Model file for the job. Use its own axes, mm. Give positions to 0.01 mm unless a question says otherwise; leave off trailing zeros. Order: outer loops, then holes, each group sorted by start corner. A loop starts at its lowest first (then second) coordinate and runs counter-clockwise, first axis right, second up. Notation, with made-up numbers: (51, 74.5) -> (109, 74.5) arc R19 ccw to (109, 84.5) -> close; hole circle Ø10 at (-22.5, 89.25). An arc over 180 degrees is marked (long way). Use CSV: the item, a comma, the result in double quotes. Start each with the question number.
1. Cut at A-A on y = 2. List the corners of the cut face in (x, z).
2. Wall check: line 1 (X direction, y = -15, z = 116.5); line 2 (Y direction, x = -28.5, z = 28); line 3 (Y direction, x = -27.5, z = 75). Give the ranges that are in metal, low to high. Write a range as from..to.
3. Drop a flat-ended pin along its axis: pin 1 (3 mm diameter, centred on x = 13.5, z = 142.5, fed in from +Y). Give the stop position or say it passes through.
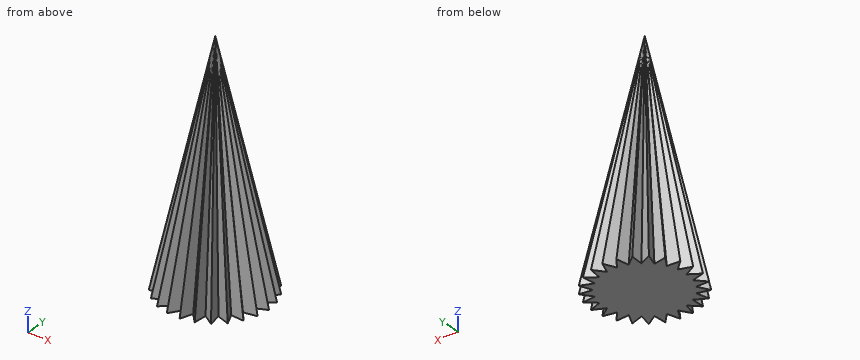
```python
from build123d import *

# Parameters (mm, degrees)
F8_COUNT = 25


with BuildPart() as f1:
    # F0 (on Front) → F1 (revolve)
    with BuildSketch(Plane.XZ):
        Polygon((-45, 0), (0, 0), (0, 200), align=None)
    revolve(axis=Axis((0, 0, 100), (0, 0, 1)))


with BuildPart() as f7:
    # F7: sweep along a path in F6
    with BuildLine(Plane.XZ) as f7_path:
        Line((-35, 0), (2.9236729855, 216.7067027743))
    # F5 (on face) → F7 (sweep)
    with BuildSketch(Plane(origin=(0, 0, 0), x_dir=(1, 0, 0), z_dir=(0, 0, -1))):
        with BuildLine():
            Line((-44.6429487171, -5.6574844095), (-35, 0))
            Line((-35, 0), (-44.6429487171, 5.6574844095))
            ThreePointArc((-44.6429487171, 5.6574844095), (-45, 0), (-44.6429487171, -5.6574844095))
        make_face()
    sweep(path=f7_path.line)


with BuildPart() as f8_1:
    # F8: instance of F7
    add(f7.part.rotate(Axis((0, 0, 0), (0, 0, 1)), 1 * 360 / F8_COUNT))


with BuildPart() as f8_2:
    # F8: instance of F7
    add(f7.part.rotate(Axis((0, 0, 0), (0, 0, 1)), 2 * 360 / F8_COUNT))


with BuildPart() as f8_3:
    # F8: instance of F7
    add(f7.part.rotate(Axis((0, 0, 0), (0, 0, 1)), 3 * 360 / F8_COUNT))


with BuildPart() as f8_4:
    # F8: instance of F7
    add(f7.part.rotate(Axis((0, 0, 0), (0, 0, 1)), 4 * 360 / F8_COUNT))


with BuildPart() as f8_5:
    # F8: instance of F7
    add(f7.part.rotate(Axis((0, 0, 0), (0, 0, 1)), 5 * 360 / F8_COUNT))


with BuildPart() as f8_6:
    # F8: instance of F7
    add(f7.part.rotate(Axis((0, 0, 0), (0, 0, 1)), 6 * 360 / F8_COUNT))


with BuildPart() as f8_7:
    # F8: instance of F7
    add(f7.part.rotate(Axis((0, 0, 0), (0, 0, 1)), 7 * 360 / F8_COUNT))


with BuildPart() as f8_8:
    # F8: instance of F7
    add(f7.part.rotate(Axis((0, 0, 0), (0, 0, 1)), 8 * 360 / F8_COUNT))


with BuildPart() as f8_9:
    # F8: instance of F7
    add(f7.part.rotate(Axis((0, 0, 0), (0, 0, 1)), 9 * 360 / F8_COUNT))


with BuildPart() as f8_10:
    # F8: instance of F7
    add(f7.part.rotate(Axis((0, 0, 0), (0, 0, 1)), 10 * 360 / F8_COUNT))


with BuildPart() as f8_11:
    # F8: instance of F7
    add(f7.part.rotate(Axis((0, 0, 0), (0, 0, 1)), 11 * 360 / F8_COUNT))


with BuildPart() as f8_12:
    # F8: instance of F7
    add(f7.part.rotate(Axis((0, 0, 0), (0, 0, 1)), 12 * 360 / F8_COUNT))


with BuildPart() as f8_13:
    # F8: instance of F7
    add(f7.part.rotate(Axis((0, 0, 0), (0, 0, 1)), 13 * 360 / F8_COUNT))


with BuildPart() as f8_14:
    # F8: instance of F7
    add(f7.part.rotate(Axis((0, 0, 0), (0, 0, 1)), 14 * 360 / F8_COUNT))


with BuildPart() as f8_15:
    # F8: instance of F7
    add(f7.part.rotate(Axis((0, 0, 0), (0, 0, 1)), 15 * 360 / F8_COUNT))


with BuildPart() as f8_16:
    # F8: instance of F7
    add(f7.part.rotate(Axis((0, 0, 0), (0, 0, 1)), 16 * 360 / F8_COUNT))


with BuildPart() as f8_17:
    # F8: instance of F7
    add(f7.part.rotate(Axis((0, 0, 0), (0, 0, 1)), 17 * 360 / F8_COUNT))


with BuildPart() as f8_18:
    # F8: instance of F7
    add(f7.part.rotate(Axis((0, 0, 0), (0, 0, 1)), 18 * 360 / F8_COUNT))


with BuildPart() as f8_19:
    # F8: instance of F7
    add(f7.part.rotate(Axis((0, 0, 0), (0, 0, 1)), 19 * 360 / F8_COUNT))


with BuildPart() as f8_20:
    # F8: instance of F7
    add(f7.part.rotate(Axis((0, 0, 0), (0, 0, 1)), 20 * 360 / F8_COUNT))


with BuildPart() as f8_21:
    # F8: instance of F7
    add(f7.part.rotate(Axis((0, 0, 0), (0, 0, 1)), 21 * 360 / F8_COUNT))


with BuildPart() as f8_22:
    # F8: instance of F7
    add(f7.part.rotate(Axis((0, 0, 0), (0, 0, 1)), 22 * 360 / F8_COUNT))


with BuildPart() as f8_23:
    # F8: instance of F7
    add(f7.part.rotate(Axis((0, 0, 0), (0, 0, 1)), 23 * 360 / F8_COUNT))


with BuildPart() as f8_24:
    # F8: instance of F7
    add(f7.part.rotate(Axis((0, 0, 0), (0, 0, 1)), 24 * 360 / F8_COUNT))


with BuildPart() as f1_1:
    add(f1.part)

    # F9: cut F7, F8_1, F8_2, F8_3, F8_6, F8_7, F8_8, F8_9, F8_10, F8_11, F8_12, F8_13, F8_14, F8_15, F8_16, F8_17, F8_18, F8_19, F8_20, F8_21, F8_22, F8_23, F8_24, F8_4, F8_5
    add(f7.part, mode=Mode.SUBTRACT)
    add(f8_1.part, mode=Mode.SUBTRACT)
    add(f8_2.part, mode=Mode.SUBTRACT)
    add(f8_3.part, mode=Mode.SUBTRACT)
    add(f8_6.part, mode=Mode.SUBTRACT)
    add(f8_7.part, mode=Mode.SUBTRACT)
    add(f8_8.part, mode=Mode.SUBTRACT)
    add(f8_9.part, mode=Mode.SUBTRACT)
    add(f8_10.part, mode=Mode.SUBTRACT)
    add(f8_11.part, mode=Mode.SUBTRACT)
    add(f8_12.part, mode=Mode.SUBTRACT)
    add(f8_13.part, mode=Mode.SUBTRACT)
    add(f8_14.part, mode=Mode.SUBTRACT)
    add(f8_15.part, mode=Mode.SUBTRACT)
    add(f8_16.part, mode=Mode.SUBTRACT)
    add(f8_17.part, mode=Mode.SUBTRACT)
    add(f8_18.part, mode=Mode.SUBTRACT)
    add(f8_19.part, mode=Mode.SUBTRACT)
    add(f8_20.part, mode=Mode.SUBTRACT)
    add(f8_21.part, mode=Mode.SUBTRACT)
    add(f8_22.part, mode=Mode.SUBTRACT)
    add(f8_23.part, mode=Mode.SUBTRACT)
    add(f8_24.part, mode=Mode.SUBTRACT)
    add(f8_4.part, mode=Mode.SUBTRACT)
    add(f8_5.part, mode=Mode.SUBTRACT)


solid = f1_1.part
```
Verdict:
1,outline,"(-38.41, 0) -> (40.29, 0) -> (15.83, 108.81) -> (7.79, 164.22) -> (5.05, 168.95) -> (3.64, 181.53) -> (2.75, 180.56) -> (2.13, 187) -> (1.65, 185.17) -> (1.27, 189.46) -> (0.94, 187.37) -> (0.65, 190.65) -> (0.38, 188.37) -> (0.13, 191.09) -> (-0.13, 188.55) -> (-0.38, 190.94) -> (-0.65, 187.98) -> (-0.94, 190.17) -> (-1.27, 186.46) -> (-1.65, 188.45) -> (-2.13, 183.3) -> (-2.75, 184.86) -> (-3.64, 176.28) -> (-5.05, 175.83) -> (-7.79, 154.04) -> (-15.83, 129.01) -> close"
2,line 1,"-7.92..-5.76, -4.27..-1.2, -0.71..2.51, 3.3..6.06, 8.82..9.92"
2,line 2,"-22.09..-18.06, -14.44..14.44, 18.06..22.09"
2,line 3,"-3.63..-3.3, 3.3..3.63"
3,pin 1,"y = 3.33"
